Part print with two shaded views. Sizes in mm from the minimum x, y, z corner. Give positions to 0.01 mm unless a question says otherwise; leave off trailing zeros. Write each loop counter-clockwise with the first axis right and the second up, starting at its lowest first coordinate (ties: lowest second). Pieces come first, ordered by that corner, then holes. Notation, with made-up numbers: (26.25, -26) -> (50.25, -26) arc R19 cw to (50.25, -13) -> close; hole circle Ø1 at (68.5, 58). An arc over 180 degrees is marked (long way). Answer as a JSON object with one key per item and string values.
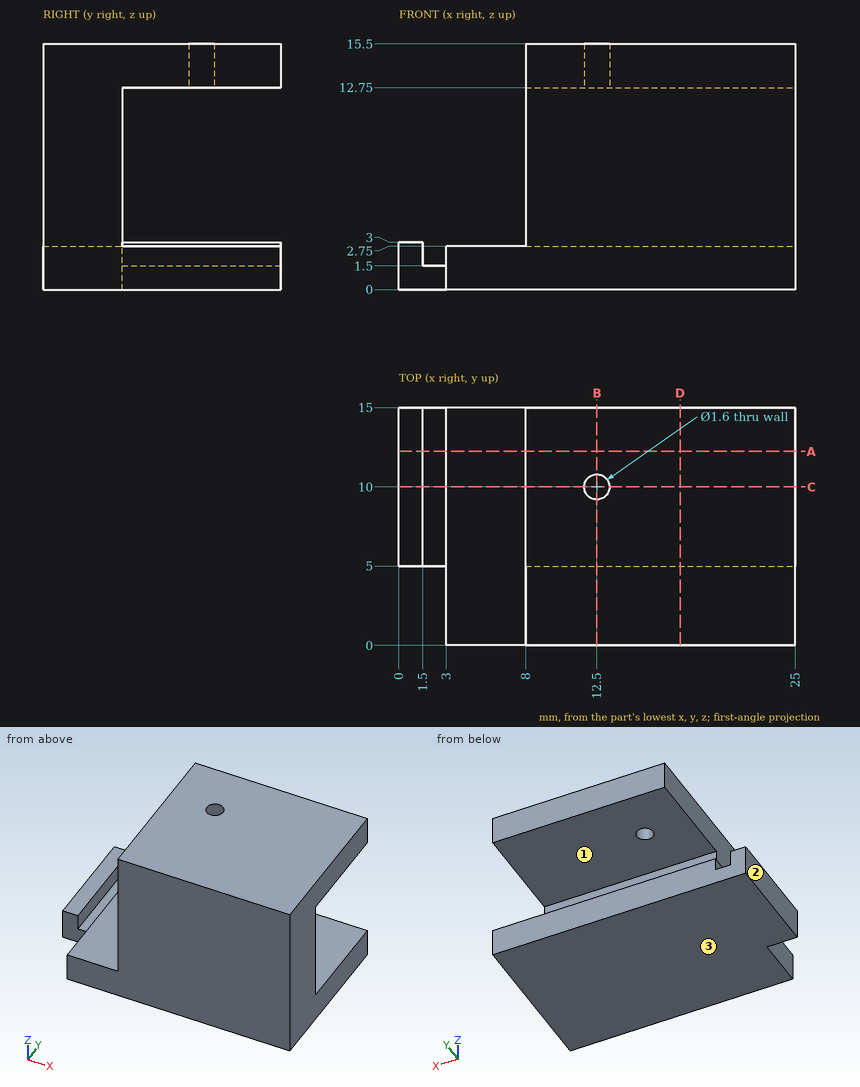
1) Slice it at D-D (x = 17.75). List the corners of the cut face in (y, z).
Model answer:
{"outline": "(0, 0) -> (15, 0) -> (15, 2.75) -> (5, 2.75) -> (5, 12.75) -> (15, 12.75) -> (15, 15.5) -> (0, 15.5) -> close"}
2) Mould opens along Z. For the marked faces 1, 2 and 3 say: released by +Z, released by -Z, zero draft, split by the parting line, or undercut.
Model answer:
{"face 1": "undercut", "face 2": "zero draft", "face 3": "released by -Z"}
3) Wall check: probe 1 along Y at (x, z) = (12.5, 14.95); probe 2 along X at (y, z) = (11, 2.25); probe 3 along Z at (x, y) = (24, 13.75). Give the ranges that are in metal, low to high.
Model answer:
{"probe 1": "y = 0 to 9.2, 10.8 to 15", "probe 2": "x = 0 to 1.5, 3 to 25", "probe 3": "z = 0 to 2.75, 12.75 to 15.5"}
4) Slice it at A-A (y = 12.25). List the corners of the cut face in (x, z), then the cut area to 3 significant figures.
Model answer:
{"outline": "(0, 0) -> (25, 0) -> (25, 2.75) -> (3, 2.75) -> (3, 1.5) -> (1.5, 1.5) -> (1.5, 3) -> (0, 3) -> close; (8, 12.75) -> (25, 12.75) -> (25, 15.5) -> (8, 15.5) -> close", "area": "114 mm2"}
5) Pin check, flat tips, straight feed: pin 1 (1.3 mm diameter, centred on x = 12.5, y = 10, fed in from +Z); pin 2 (4 mm diameter, centred on y = 10.5, z = 10.5, fed in from -X); pin 3 (0.9 mm diameter, centred on x = 1.5, z = 1, fed in from -Y); pin 4 (8 mm diameter, centred on x = 17.5, z = 3.5, fed in from -Y). Stop position of each tip, or through.
Model answer:
{"pin 1": "stops at z = 2.75", "pin 2": "passes through", "pin 3": "stops at y = 5", "pin 4": "stops at y = 0"}
6) Slice it at B-B (x = 12.5). List the corners of the cut face in (y, z).
Model answer:
{"outline": "(0, 0) -> (15, 0) -> (15, 2.75) -> (5, 2.75) -> (5, 12.75) -> (9.2, 12.75) -> (9.2, 15.5) -> (0, 15.5) -> close; (10.8, 12.75) -> (15, 12.75) -> (15, 15.5) -> (10.8, 15.5) -> close"}
7) Slice it at C-C (y = 10). List the corners of the cut face in (x, z), then the cut area to 3 significant figures.
Model answer:
{"outline": "(0, 0) -> (25, 0) -> (25, 2.75) -> (3, 2.75) -> (3, 1.5) -> (1.5, 1.5) -> (1.5, 3) -> (0, 3) -> close; (8, 12.75) -> (11.7, 12.75) -> (11.7, 15.5) -> (8, 15.5) -> close; (13.3, 12.75) -> (25, 12.75) -> (25, 15.5) -> (13.3, 15.5) -> close", "area": "110 mm2"}
